Study the drawing (mm; zero at the part's minimum x, y, z) and answer. A direction names the side the tool comes from. Coordinates: 2 decimals unless noted, no trailing zeros. Order: outer loops, then holes, each group sorted by start corner. A loop starts at its lowest first (then second) coordinate and runs counter-clockwise, first axis right, second up. Notation, with made-up numbers: M 75,33.5 L 84,33.5 A11 cw 84,47.5 Z; hole C 65.25,80.25 d7. An arc over 180 degrees is marked long. One line per item, written item: value. Start each with the question number.
Q1. The part is cut by section B-B on y = 8. Give the vertices of the cut face in (x, z), then the cut area to 3 significant figures.
Q2. The part is cut by section C-C on x = 25.5. Give the vertices of the cut face in (y, z), then the cut area to 3 significant figures.
Q3. Each of these flat-tipped pins is pushed along its axis until it touches: pin 1 Ø8 at (y, z) = (6, 22.5) entering from +X; pin 2 Ø6.5 at (x, y) = (15, 6) entering from -Z; pin 3 Ø5 at (x, y) = (19.5, 6) entering from +Z; pin 4 Ø5 at (y, z) = (7, 29) entering from +X. Where does it stop, or does it pass through?
Q4. The part is cut by section A-A on z = 21. Give the vertices of the cut face in (x, y), then the cut area to 3 significant figures.
Q5. The part is cut by section D-D on z = 25. Give the vertices of the cut face in (x, y), then the cut area to 3 significant figures.
Q6. Determine the mould class of the marked faces 1, 2 and 3 for opening direction X: pulls with the +X half, pulls with the -X half, needs draft (parallel to the pull), parting line crosses it, or undercut.
Q7. For the marked faces 4, 5 and 6, determine the directions among +Z, -Z, +X, -X, +Y, -Y from which every point of the face is accessible in a straight line to the end or side of a thin tool.
Q8. Straight lines are drawn through the part: line 1 along Z through (x, y) = (15, 13.4); line 2 along Y through (x, z) = (6, 29.5); line 3 along Z through (x, y) = (15.5, 10.25). For each, find the intervals that lie inside material, in ascending order. Write a range as [from, to].
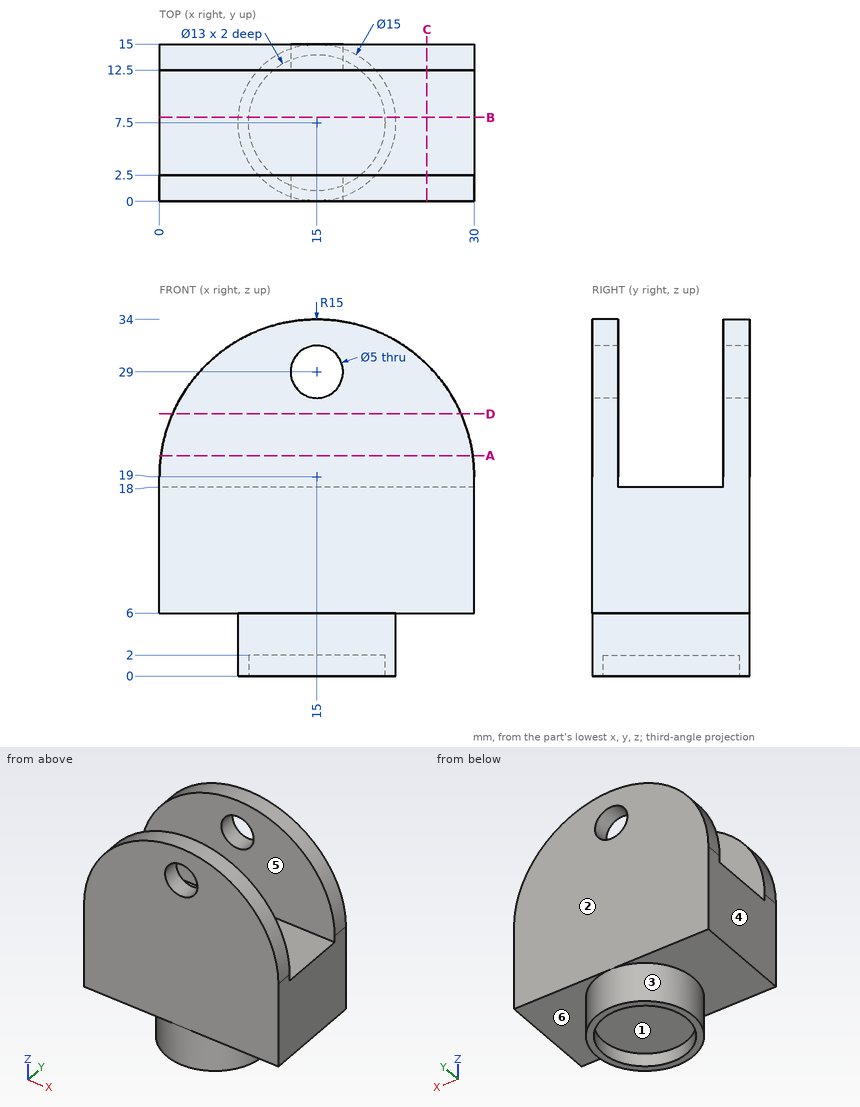
Output:
1. outline: M 0,6 L 7.52,6 L 7.52,0 L 8.52,0 L 8.52,2 L 21.48,2 L 21.48,0 L 22.48,0 L 22.48,6 L 30,6 L 30,18 L 0,18 Z
1. area: 424 mm^2
2. outline: M 0,6 L 15,6 L 15,29.71 L 12.5,29.71 L 12.5,18 L 2.5,18 L 2.5,29.71 L 0,29.71 Z
2. area: 239 mm^2
3. pin 1: stops at x = 29.92
3. pin 2: stops at z = 2
3. pin 3: stops at z = 18
3. pin 4: passes through
4. outline: M 0.13,0 L 29.87,0 L 29.87,2.5 L 0.13,2.5 Z; M 0.13,12.5 L 29.87,12.5 L 29.87,15 L 0.13,15 Z
4. area: 149 mm^2
5. outline: M 1.25,0 L 28.75,0 L 28.75,2.5 L 1.25,2.5 Z; M 1.25,12.5 L 28.75,12.5 L 28.75,15 L 1.25,15 Z
5. area: 137 mm^2
6. face 1: undercut
6. face 2: needs draft
6. face 3: parting line crosses it
7. face 4: +Z, -Z, -X, +Y, -Y
7. face 5: +Z, +X, -X
7. face 6: -Z, +X
8. line 1: z = [2, 26.5], [31.5, 34]
8. line 2: y = [0, 2.5], [12.5, 15]
8. line 3: z = [2, 18]
